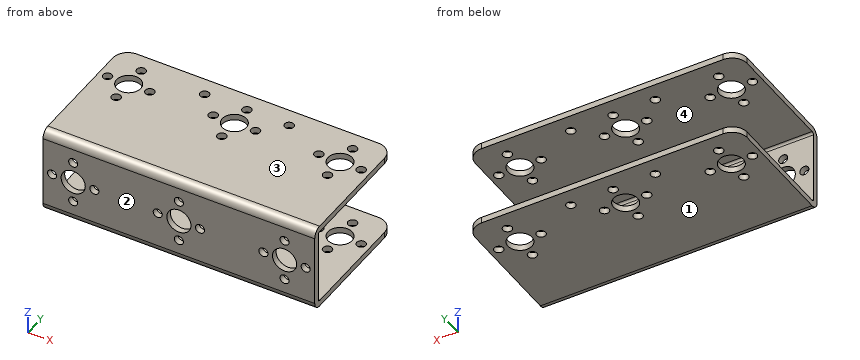
```python
from build123d import *

# Parameters (mm, degrees)
SKETCH_1_W                         = 90
SKETCH_1_H                         = 29
SKETCH_1_R                         = 4
SKETCH_1_R_2                       = 1.5
SM_BASE_FLANGE_1_DEPTH             = 2
SM_EDGE_FLANGE_1_STRIP_W           = 9.4732
SM_EDGE_FLANGE_1_STRIP_H           = 2
SM_EDGE_FLANGE_1_STRIP_CUT_DEPTH   = 90
SM_EDGE_FLANGE_1_STRIP_2_W         = 9.4732
SM_EDGE_FLANGE_1_STRIP_2_H         = 2
SM_EDGE_FLANGE_1_STRIP_CUT_2_DEPTH = 90
SM_EDGE_FLANGE_1_DEPTH             = 90
SM_EDGE_FLANGE_1_BEND_DEPTH        = 90
SKETCH_12_R                        = 4
SKETCH_12_R_2                      = 1.5
CUT_EXTRUDE_1_DEPTH                = 55
FILLET_1_R                         = 5


# Sheet-metal steps are written as plain solids
with BuildPart() as part:
    # Sketch 1 → 基体-法兰1 (new body)
    with BuildSketch(Plane(origin=(0, 0, 0), x_dir=(1, 0, 0), z_dir=(0, 1, 0))):
        with Locations((45, -14.5)):
            Rectangle(SKETCH_1_W, SKETCH_1_H)
        with Locations(Location((45, -14.5, 0), (0, 0, 270))):
            Circle(SKETCH_1_R, mode=Mode.SUBTRACT)
        with Locations(Location((10, -14.5, 0), (0, 0, 270))):
            Circle(SKETCH_1_R, mode=Mode.SUBTRACT)
        with Locations(Location((80, -14.5, 0), (0, 0, 270))):
            Circle(SKETCH_1_R, mode=Mode.SUBTRACT)
        with Locations(Location((10, -7.5, 0), (0, 0, 270))):
            Circle(SKETCH_1_R_2, mode=Mode.SUBTRACT)
        with Locations(Location((10, -21.5, 0), (0, 0, 270))):
            Circle(SKETCH_1_R_2, mode=Mode.SUBTRACT)
        with Locations(Location((17, -14.5, 0), (0, 0, 270))):
            Circle(SKETCH_1_R_2, mode=Mode.SUBTRACT)
        with Locations(Location((3, -14.5, 0), (0, 0, 270))):
            Circle(SKETCH_1_R_2, mode=Mode.SUBTRACT)
        with Locations(Location((45, -7.5, 0), (0, 0, 270))):
            Circle(SKETCH_1_R_2, mode=Mode.SUBTRACT)
        with Locations(Location((45, -21.5, 0), (0, 0, 270))):
            Circle(SKETCH_1_R_2, mode=Mode.SUBTRACT)
        with Locations(Location((52, -14.5, 0), (0, 0, 270))):
            Circle(SKETCH_1_R_2, mode=Mode.SUBTRACT)
        with Locations(Location((38, -14.5, 0), (0, 0, 270))):
            Circle(SKETCH_1_R_2, mode=Mode.SUBTRACT)
        with Locations(Location((87, -14.5, 0), (0, 0, 90))):
            Circle(SKETCH_1_R_2, mode=Mode.SUBTRACT)
        with Locations(Location((80, -21.5, 0), (0, 0, 90))):
            Circle(SKETCH_1_R_2, mode=Mode.SUBTRACT)
        with Locations(Location((73, -14.5, 0), (0, 0, 90))):
            Circle(SKETCH_1_R_2, mode=Mode.SUBTRACT)
        with Locations(Location((80, -7.5, 0), (0, 0, 90))):
            Circle(SKETCH_1_R_2, mode=Mode.SUBTRACT)
    extrude(amount=-SM_BASE_FLANGE_1_DEPTH)

    # 边线-法兰1 strip (across the edge) → 边线-法兰1 strip cut (cut)
    with BuildSketch(Plane.ZY.offset(-90)):
        with Locations((-2, -1)):
            Rectangle(SM_EDGE_FLANGE_1_STRIP_W, SM_EDGE_FLANGE_1_STRIP_H)
    extrude(amount=SM_EDGE_FLANGE_1_STRIP_CUT_DEPTH, mode=Mode.SUBTRACT)

    # 边线-法兰1 strip 2 (across the edge) → 边线-法兰1 strip cut 2 (cut)
    with BuildSketch(Plane(origin=(0, 0, 29), x_dir=(0, 0, -1), z_dir=(1, 0, 0))):
        with Locations((-2, -1)):
            Rectangle(SM_EDGE_FLANGE_1_STRIP_2_W, SM_EDGE_FLANGE_1_STRIP_2_H)
    extrude(amount=SM_EDGE_FLANGE_1_STRIP_CUT_2_DEPTH, mode=Mode.SUBTRACT)

    # 边线-法兰1 section (across the edge) → 边线-法兰1 (add)
    with BuildSketch(Plane.ZY.offset(-90)):
        with BuildLine():
            Line((0, 0.7366), (0, 42))
            Line((0, 42), (2, 42))
            Line((2, 42), (2, 0.7366))
            ThreePointArc((2, 0.7366), (2.215745145, 0.215745145), (2.7366, 0))
            Line((2.7366, 0), (2.7366, -2))
            ThreePointArc((2.7366, -2), (0.801531583, -1.198468417), (0, 0.7366))
        make_face()
    extrude(amount=SM_EDGE_FLANGE_1_DEPTH)

    # 边线-法兰1 section 2 (across the edge) → 边线-法兰1 bend (add)
    with BuildSketch(Plane(origin=(0, 0, 29), x_dir=(0, 0, -1), z_dir=(1, 0, 0))):
        with BuildLine():
            Line((0, 0.7366), (0, 42))
            Line((0, 42), (2, 42))
            Line((2, 42), (2, 0.7366))
            ThreePointArc((2, 0.7366), (2.215745145, 0.215745145), (2.7366, 0))
            Line((2.7366, 0), (2.7366, -2))
            ThreePointArc((2.7366, -2), (0.801531583, -1.198468417), (0, 0.7366))
        make_face()
    extrude(amount=SM_EDGE_FLANGE_1_BEND_DEPTH)

    # 草图12 → 切除-拉伸1 (cut)
    with BuildSketch(Plane.XY.offset(29)):
        with Locations((45, 29)):
            Circle(SKETCH_12_R)
        with Locations((80, 29)):
            Circle(SKETCH_12_R)
        with Locations((10, 29)):
            Circle(SKETCH_12_R)
        with Locations((10, 36)):
            Circle(SKETCH_12_R_2)
        with Locations((10, 22)):
            Circle(SKETCH_12_R_2)
        with Locations((17, 29)):
            Circle(SKETCH_12_R_2)
        with Locations((3, 29)):
            Circle(SKETCH_12_R_2)
        with Locations((45, 36)):
            Circle(SKETCH_12_R_2)
        with Locations((45, 22)):
            Circle(SKETCH_12_R_2)
        with Locations((52, 29)):
            Circle(SKETCH_12_R_2)
        with Locations((38, 29)):
            Circle(SKETCH_12_R_2)
        with Locations(Location((87, 29, 0), (0, 0, 90))):
            Circle(SKETCH_12_R_2)
        with Locations(Location((80, 36, 0), (0, 0, 90))):
            Circle(SKETCH_12_R_2)
        with Locations(Location((73, 29, 0), (0, 0, 90))):
            Circle(SKETCH_12_R_2)
        with Locations(Location((80, 22, 0), (0, 0, 90))):
            Circle(SKETCH_12_R_2)
        with Locations((31, 36)):
            Circle(SKETCH_12_R_2)
        with Locations((59, 36)):
            Circle(SKETCH_12_R_2)
    extrude(amount=-CUT_EXTRUDE_1_DEPTH, mode=Mode.SUBTRACT)

    # 圆角1
    fillet_1_edges = [part.edges().sort_by_distance(p)[0] for p in [
        (90, 42, 1),
        (0, 42, 1),
        (0, 42, 28),
        (90, 42, 28),
    ]]
    fillet(fillet_1_edges, radius=FILLET_1_R)


solid = part.part
```
Input: part model. Units: mm. Frame: model coordinates. Face numbers are marked on the shaded views. Round coordinates to 2 decimals unless told otherwise and drop trailing zeros. Loops run counter-clockwise (first coordinate to the right, second up) from the corner with the lowest first, then second, coordinate; pieces in that order, holes last. Notation, with made-up numbers: M 13.5,29.5 L 20.5,29.5 A27 ccw 20.5,56.5 Z; hole C 82,-5.5 d1. An arc over 180 degrees is marked long. Answer in a Markdown table with one row per item. Add a question column.
1. Section A-A (x = 52). Output: boundary loops of the cut face in (y, z).
2. Mould query, pull axis Z, two halves, no side actions, for the marked faces 1, 2, 3 and 4. Classes: released by +Z, released by -Z, zero draft, split by the parting line, or undercut.
3. Section C-C (y = 39.5). Output: boundary loops of the cut face in (x, z).
4. Contact query for flat-ended pins moving along their axis: pin 1 (1.8 mm diameter, centred on x = 45, z = 21.5, fed in from -Y); pin 2 (3 mm diameter, centred on x = 30.5, z = 14, fed in from +Y). Output: stop coordinate, or through.
5. Section B-B (z = 7.5). Output: boundary loops of the cut face in (x, y), and give its area (3 significant figures).
6. Ray query, probe 1 along Z at (x, y) = (73, 22.5); probe 2 along Y at (x, z) = (10, 0.65); probe 3 along Y at (x, z) = (10, 27.6). Return the intervals inside material, ascending.
7. Section D-D (y = 22). Give the number of separate pieces and of enclosed holes in the cut face, and give its area (3 significant figures).
Values follow:
| question | item | result |
|---|---|---|
| 1 | outline | M -2,2.74 A2.74 ccw 0.74,0 L 27.5,0 L 27.5,2 L 0.74,2 A0.74 cw 0,2.74 L 0,13 L -2,13 Z; M -2,16 L 0,16 L 0,26.26 A0.74 cw 0.74,27 L 27.5,27 L 27.5,29 L 0.74,29 A2.74 ccw -2,26.26 Z; M 30.5,0 L 42,0 L 42,2 L 30.5,2 Z; M 30.5,27 L 42,27 L 42,29 L 30.5,29 Z |
| 2 | face 1 | released by -Z |
| 2 | face 2 | zero draft |
| 2 | face 3 | released by +Z |
| 2 | face 4 | undercut |
| 3 | outline | M 0.67,0 L 89.33,0 L 89.33,2 L 0.67,2 Z; M 0.67,27 L 89.33,27 L 89.33,29 L 0.67,29 Z |
| 4 | pin 1 | through |
| 4 | pin 2 | y = 0 |
| 5 | outline | M 0,-2 L 8.5,-2 L 8.5,0 L 0,0 Z; M 11.5,-2 L 43.5,-2 L 43.5,0 L 11.5,0 Z; M 46.5,-2 L 78.5,-2 L 78.5,0 L 46.5,0 Z; M 81.5,-2 L 90,-2 L 90,0 L 81.5,0 Z |
| 5 | area | 162 mm^2 |
| 6 | probe 1 | 0 to 2, 27 to 29 |
| 6 | probe 2 | -1.03 to 20.5, 23.5 to 25, 33 to 34.5, 37.5 to 42 |
| 6 | probe 3 | -1.65 to 20.5, 23.5 to 25, 33 to 34.5, 37.5 to 42 |
| 7 | separate pieces | 8 |
| 7 | enclosed holes | 0 |
| 7 | area | 324 mm^2 |
